Design review of the part built by this model. Coordinates are the model's own, in mm. A direction names the side the tool comes from. Round coordinates to 2 decimals unless told otherwise and drop trailing zeros. Loops run counter-clockwise (first coordinate to the right, second up) from the corner with the lowest first, then second, coordinate; pieces in that order, holes last. Notation, with made-up numbers: (10.5, 73.5) - (23.5, 73.5) arc R24 ccw to (23.5, 110.5) - close; hole circle Ø8 at (86, 83). An arc over 180 degrees is marked (long way). Return JSON: item names as keys, results as strings. Group by question number.
Autodesk Fusion 360 part; units mm, degrees
sketch "Sketch1" plane through (0, 0, 0) normal (1, 0, 0) x (0, 1, 0)
  circle A0 centre (0, 0) radius 51
  dimension "d1" = 102
extrude "Extrude1" add sketch "Sketch1" along normal blind 32 makes body 1
sketch "Sketch2" plane through (32, 0, 0) normal (1, 0, 0) x (0, 1, 0)
  circle A0 centre (0, 0) radius 51
  circle A1 centre (0, 0) radius 51
  line L0 (-56, 0) -> (56, 0)
  line L1 (56, 0) -> (56, -61)
  line L2 (56, -61) -> (-56, -61)
  line L3 (-56, -61) -> (-56, 0)
  dimension "d5" = 5
  dimension "d6" = 5
  dimension "d7" = 10
extrude "Extrude2" add sketch "Sketch2" against normal blind 15 separate body contours A0 A1 L0 L1 L2 L3 makes body 2
combine "Combine1" operation cut target body 2 tool bodies 1
sketch "Sketch3" plane through (0, 0, 0) normal (0, 0, 1) x (1, 0, 0)
  line L0 (32, -56) -> (17, -56)
  line L1 (32, 56) -> (17, 56)
  line L2 (32, 51) -> (17, 51)
  line L3 (17, 56) -> (17, 51)
  line L4 (32, 51) -> (32, 56)
  line L5 (32, -56) -> (32, -51)
  line L6 (17, -51) -> (17, -56)
  line L7 (32, -51) -> (17, -51)
  line L8 (32, -51) -> (32, 51) construction
  line L9 (17, -51) -> (17, 51) construction
  line L10 (32, 0) -> (0, 0) construction
  line L11 (62, -12.5) -> (32, -12.5)
  line L12 (32, -12.5) -> (32, 12.5)
  line L13 (32, 12.5) -> (62, 12.5)
  line L14 (62, 12.5) -> (62, -12.5)
  line L15 (62, 0) -> (32, 0) construction
  circle A0 centre (54.25, 0) radius 2.75
  circle A1 centre (54.25, 0) radius 1.5
  line L16 (24.5, 56) -> (24.5, 51) construction
  line L17 (37, 56) -> (12, 56)
  line L18 (12, 56) -> (12, 86)
  line L19 (12, 86) -> (37, 86)
  line L20 (37, 86) -> (37, 56)
  line L21 (24.5, 56) -> (24.5, 86) construction
  circle A2 centre (24.5, 78.25) radius 2.75
  circle A3 centre (24.5, 78.25) radius 1.5
  point P0 (32, 56)
  point P1 (54.25, 0)
  dimension "d10" = 30
  dimension "d11" = 25
  dimension "d12" = 5.5
  dimension "d13" = 3
  dimension "d14" = 5
  dimension "d29" = 5.5
  dimension "d30" = 5
  dimension "d31" = 3
extrude "Extrude5" add sketch "Sketch3" along normal blind 10 from surface at -61 contours L1 L17 L18 L19 L20 | A2 bodies 2
extrude "Extrude6" cut sketch "Sketch3" against normal blind 5 from surface at -51 contours A2 bodies 2
move_face "OffsetFaces2" offset 15 2 faces at (27, -54.3333, 0) (27, 52.6667, 0) on bodies 2
fillet "Fillet4" radius 5 2 edges at (37, 86, -56) (12, 86, -56) on bodies 2
fillet "Fillet6" radius 60 1 edges at (24.5, -56, -61) on bodies 2
fillet "Fillet7" radius 3 2 edges at (12, 56, -56) (37, 56, -56) on bodies 2
chamfer "Chamfer2" distance 15 angle 45 1 edges at (24.5, 56, -51) on bodies 2
Q1. Add section B-B, the plane z = 1.5. State the section outline as (x, y) points.
Q2. Tool access review of faces 1 (the flat face through (25, -52, 15)), 2 (the flat face through (25, 56, -10)): name each direction out of +Z, -Z, +X, -X, +Y, -Y from which nothing blocks a thin tool from reaching the whole face with its end or side.
Q3. For line 1 (Y direction, x = 22, z = 1); line 2 (Y direction, x = 29.25, z = -34.5); line 3 (X direction, y = -45.5, z = -27), list the stretches that pass through material, from the lowest coordinate up.
Q4. Add section C-C, the plane x = 24.5. State the section outline as (y, z) points, plus the area to 3 significant figures.
Q5. Add section D-D, the plane y = 0. State the section outline as (x, z) points, plus the area to 3 significant figures.
Q6. Insertion check: pin 1 Ø5 at (x, z) = (26.5, -32) entering from -Y; pin 2 Ø0.6 at (x, z) = (16.5, -57.5) entering from -Y; pin 3 Ø3 at (x, y) = (24, 78) entering from +Z. Each pin has a flat end and moves straight along its axis. Give the tip position at first contact, or say it passes through.
Q7. Draft analysis for pull direction X (two halves, no side actions). For faces 3 (the flat face through (26, 77, -56)), 4 (the cylindrical face through (14, 85, -56)), 5 (the flat face through (24, 75, -51)), state which applies: pulls with the +X half, pulls with the -X half, needs draft (parallel to the pull), parting line crosses it, or undercut.
Q8. Add section A-A, the plane y = 78.25. State the section outline as (x, z) points.
Evaluation:
{
 "1": {"outline": "(17, -56) - (32, -56) - (32, -50.98) - (17, -50.98) - close; (17, 50.98) - (32, 50.98) - (32, 56) - (17, 56) - close"},
 "2": {"face 1": "+Z, +X, -X, +Y, -Y", "face 2": "+Z, +X, -X, +Y"},
 "3": {"line 1": "-56 to -50.99, 50.99 to 56", "line 2": "-45.78 to -37.56, 37.56 to 56", "line 3": "17 to 32"},
 "4": {"outline": "(-56, -1) arc R60 ccw to (4, -61) - (76.75, -61) - (76.75, -56) - (75.5, -56) - (75.5, -51) - (71, -51) - (56, -36) - (56, 15) - (48.74, 15) arc R51 cw (long way) to (-48.74, 15) - (-56, 15) - close; (79.75, -61) - (86, -61) - (86, -51) - (81, -51) - (81, -56) - (79.75, -56) - close", "area": "2,520 mm²"},
 "5": {"outline": "(17, -60.87) - (32, -60.87) - (32, -51) - (17, -51) - close", "area": "148 mm²"},
 "6": {"pin 1": "y = -48.8", "pin 2": "y = 56", "pin 3": "z = -56"},
 "7": {"face 3": "undercut", "face 4": "pulls with the -X half", "face 5": "needs draft"},
 "8": {"outline": "(12, -61) - (23, -61) - (23, -56) - (21.75, -56) - (21.75, -51) - (12, -51) - close; (26, -61) - (37, -61) - (37, -51) - (27.25, -51) - (27.25, -56) - (26, -56) - close"}
}
